Read the model definition and answer for the solid it produces. Units are mm, in the model's axes. A direction names the side the tool comes from. Coordinates: 2 decimals unless noted, no trailing zeros. Order: outer loops, then holes, each group sorted by start corner. A loop starts at its lowest first (then second) coordinate and runs counter-clockwise, first axis right, second up.
```python
from build123d import *

# Parameters (mm, degrees)
F0_W     = 5
F0_H     = 5
F0_W_2   = 3
F0_H_2   = 20
F0_W_3   = 10
F1_DEPTH = 14
F2_W     = 10
F2_H     = 20
F3_DEPTH = 3
F4_R     = 5
F5_R     = 5
F6_R     = 2.49999
F7_R     = 2.49999
F8_R     = 2.5
F9_DEPTH = 25


# Not quite as in the source:
# - a fillet or chamfer is up to 0.001 mm smaller than in the source, because OpenCascade refuses the exact size


with BuildPart() as f1:
    # F0 (on Top) → F1 (new body)
    with BuildSketch(Plane.XY):
        Polygon((0, 20), (0, 0), (20, 0), (20, 20), (20, 40), (20, 60), (0, 60), (0, 40), align=None)
        with Locations((10, 10)):
            Rectangle(F0_W, F0_H, mode=Mode.SUBTRACT)
        with Locations((10, 50)):
            Rectangle(F0_W, F0_H, mode=Mode.SUBTRACT)
        with Locations((-1.5, 30)):
            Rectangle(F0_W_2, F0_H_2)
        with Locations((25, 30)):
            Rectangle(F0_W_3, F0_H_2)
    extrude(amount=F1_DEPTH)

    # F2 (on face) → F3 (join)
    with BuildSketch(Plane(origin=(0, 0, 0), x_dir=(1, 0, 0), z_dir=(0, 0, -1))):
        with Locations((25, -30)):
            Rectangle(F2_W, F2_H)
    extrude(amount=F3_DEPTH)

    # F4
    f4_edges = [f1.edges().sort_by_distance(p)[0] for p in [
        (20, 40, 7),
    ]]
    fillet(f4_edges, radius=F4_R)

    # F5
    f5_edges = [f1.edges().sort_by_distance(p)[0] for p in [
        (20, 20, 7),
    ]]
    fillet(f5_edges, radius=F5_R)

    # F6 (radius 2.5 in the source; OpenCascade refuses exactly that, so slightly less here)
    f6_edges = [f1.edges().sort_by_distance(p)[0] for p in [
        (7.5, 7.5, 7),
        (7.5, 12.5, 7),
        (12.5, 12.5, 7),
        (12.5, 7.5, 7),
    ]]
    fillet(f6_edges, radius=F6_R)

    # F7 (radius 2.5 in the source; OpenCascade refuses exactly that, so slightly less here)
    f7_edges = [f1.edges().sort_by_distance(p)[0] for p in [
        (12.5, 47.5, 7),
        (7.5, 47.5, 7),
        (7.5, 52.5, 7),
        (12.5, 52.5, 7),
    ]]
    fillet(f7_edges, radius=F7_R)

    # F8 (on face) → F9 (cut)
    with BuildSketch(Plane.XY.offset(14)):
        with Locations((25, 30)):
            Circle(F8_R)
    extrude(amount=-F9_DEPTH, mode=Mode.SUBTRACT)


solid = f1.part
```
1) A cutting plane is placed at B-B, the plane z = 1.5. State how many separate pieces and enclosed holes the cut face has, and give its area (3 significant figures).
A:
separate pieces: 1
enclosed holes: 3
area: 1,410 mm2
2) Straight lines are drawn through the part: line 1 (Z direction, x = 0.5, y = 25.5); line 2 (X direction, y = 3.5, z = 13.25); line 3 (X direction, y = 32, z = 13.5). For each, find the intervals that lie inside material, in ascending order.
A:
line 1: z = 0 to 14
line 2: x = 0 to 20
line 3: x = -3 to 23.5, 26.5 to 30
3) Flat-ended cylindrical pins translate along their axes: pin 1 Ø7 at (y, z) = (12, 7.5) entering from -X; pin 2 Ø5 at (x, z) = (27, 5) entering from +Y; pin 3 Ø2 at (x, z) = (22.5, 9.5) entering from -Y. Find the tip coordinate at first contact, or state that the pin passes through.
A:
pin 1: stops at x = 0
pin 2: stops at y = 40.03
pin 3: stops at y = 18.57
4) A cutting plane is placed at A-A, the plane y = 30. Determine the outline of the cut face in (x, z), and give its area (3 significant figures).
A:
outline: (-3, 0) - (20, 0) - (20, -3) - (22.5, -3) - (22.5, 14) - (-3, 14) - close; (27.5, -3) - (30, -3) - (30, 14) - (27.5, 14) - close
area: 407 mm2
5) Which of the six approach directions +Z, -Z, +X, -X, +Y, -Y give full straight-line access (tool end or side, diameter ignored) to faces 1 (the flat face through (27, 20, 4)), 2 (the flat face through (-2, 40, 7)), 3 (the flat face through (0, 10, 7)), 4 (the flat face through (30, 30, 6)), 5 (the cylindrical face through (11.748, 8.213, 7.098))?
A:
face 1: -Z, +X, -Y
face 2: +Z, -Z, -X, +Y
face 3: +Z, -Z, -X, -Y
face 4: +Z, -Z, +X, +Y, -Y
face 5: +Z, -Z
6) A cutting plane is placed at C-C, the plane x = 5. Determine the outline of the cut face in (y, z).
A:
outline: (0, 0) - (60, 0) - (60, 14) - (0, 14) - close
7) Determine the mould class of faces 6 (the flat face through (-2, 20, 7)), 7 (the flat face through (-3, 30, 7)), 8 (the cylindrical face through (8.213, 51.748, 7.098)), 9 (the cylindrical face through (8.213, 11.748, 7.098)) for opening direction Y: pulls with the +Y half, pulls with the -Y half, needs draft (parallel to the pull), parting line crosses it, or undercut.
A:
face 6: pulls with the -Y half
face 7: needs draft
face 8: undercut
face 9: undercut
